from build123d import *

# Parameters (mm, degrees)
SKIZZE1_R                       = 6
AUFSATZ_LINEAR_AUSTRAGEN1_DEPTH = 5.5
SKIZZE2_R                       = 9
AUFSATZ_LINEAR_AUSTRAGEN2_DEPTH = 1
SKIZZE3_R                       = 2.5
SCHNITT_LINEAR_AUSTRAGEN1_DEPTH = 19.193405399
FASE1_SIZE                      = 0.2


with BuildPart() as part:
    # Skizze1 → Aufsatz-Linear austragen1 (new, symmetric)
    with BuildSketch(Plane.XY):
        Circle(SKIZZE1_R)
    extrude(amount=AUFSATZ_LINEAR_AUSTRAGEN1_DEPTH, both=True)

    # Skizze2 → Aufsatz-Linear austragen2 (add)
    with BuildSketch(Plane.XY.offset(5.5)):
        Circle(SKIZZE2_R)
    aufsatz_linear_austragen2 = extrude(amount=AUFSATZ_LINEAR_AUSTRAGEN2_DEPTH)

    # Spiegeln1: Aufsatz-Linear austragen2 across plane
    add(aufsatz_linear_austragen2.mirror(Plane.XY))

    # Skizze3 → Schnitt-Linear austragen1 (cut, through all)
    with BuildSketch(Plane(origin=(0, 0, -6.5), x_dir=(-1, 0, 0), z_dir=(0, 0, -1))):
        Circle(SKIZZE3_R)
    extrude(amount=-SCHNITT_LINEAR_AUSTRAGEN1_DEPTH, mode=Mode.SUBTRACT)

    # Fase1
    fase1_edges = [part.edges().sort_by_distance(p)[0] for p in [
        (-9, 0, -5.5),
        (2.5, 0, 6.5),
        (2.5, 0, -6.5),
        (-9, 0, 5.5),
        (-9, 0, 6.5),
        (-9, 0, -6.5),
    ]]
    chamfer(fase1_edges, length=FASE1_SIZE)


solid = part.part
The model under review builds one solid part; all positions refer to its coordinate system, in mm. A direction names the side the tool comes from. Round coordinates to 2 decimals unless told otherwise and drop trailing zeros. Order: outer loops, then holes, each group sorted by start corner. A loop starts at its lowest first (then second) coordinate and runs counter-clockwise, first axis right, second up. Notation, with made-up numbers: (-11.75, 5) -> (12.25, 5) arc R12 cw to (12.25, 11) -> close; hole circle Ø10 at (11.5, -11.75). An arc over 180 degrees is marked (long way). Write item = value, one per line. Start each with the question number.
Item 1: For faces 4 (the face through (-2.1, 2.1, 6.5)), 5 (the face through (2, -6, -5.5)), list the 3-axis set-ups (+Z, -Z, +X, -X, +Y, -Y) from which the entire face can be reached by the end or side of a thin tool; tool diameter is ignored.
Item 2: Consider section C-C on z = -4.5. Write out the cut boundary in (x, y).
Item 3: For line 1 along Z through (x, y) = (4.75, -4.75); line 2 along Y through (x, z) = (0, -2.75); line 3 along X through (y, z) = (0.75, 6), list the stretches that pass through material, from the lowest coordinate up.
Item 4: Consider section A-A on y = 0. Write out the cut boundary in (x, z), plus the area to 3 significant figures.
Item 5: Clearance check with flat-ended pins moving along their axes: pin 1 Ø1.5 at (x, z) = (-5.5, 1) entering from +Y; pin 2 Ø1.5 at (x, z) = (-1, -5) entering from -Y; pin 3 Ø1.5 at (y, z) = (-1.5, -5) entering from -X. State where each tip first meets the part, or that it passes through.
Item 6: Mouldability with a two-part tool opening along Y and no side actions: class faces 1 (the face through (0.54, -2.44, -0.09)), 2 (the face through (-6, 0, 0)), 3 (the face through (2, -6, 5.5)) as released by +Y, released by -Y, zero draft, split by the parting line, or undercut.
Conclusion:
q1.face_4 = +Z, +X, -X, +Y, -Y
q1.face_5 = none
q2.outline = circle Ø12 at (0, 0); hole circle Ø5 at (0, 0)
q3.line_1 = -6.5 to -5.5, 5.5 to 6.5
q3.line_2 = -6 to -2.5, 2.5 to 6
q3.line_3 = -8.97 to -2.38, 2.38 to 8.97
q4.outline = (-9, -6.3) -> (-8.8, -6.5) -> (-2.7, -6.5) -> (-2.5, -6.3) -> (-2.5, 6.3) -> (-2.7, 6.5) -> (-8.8, 6.5) -> (-9, 6.3) -> (-9, 5.7) -> (-8.8, 5.5) -> (-6, 5.5) -> (-6, -5.5) -> (-8.8, -5.5) -> (-9, -5.7) -> close; (2.5, -6.3) -> (2.7, -6.5) -> (8.8, -6.5) -> (9, -6.3) -> (9, -5.7) -> (8.8, -5.5) -> (6, -5.5) -> (6, 5.5) -> (8.8, 5.5) -> (9, 5.7) -> (9, 6.3) -> (8.8, 6.5) -> (2.7, 6.5) -> (2.5, 6.3) -> close
q4.area = 103 mm2
q5.pin_1 = 3.67
q5.pin_2 = -8.97
q5.pin_3 = -8.92
q6.face_1 = undercut
q6.face_2 = split by the parting line
q6.face_3 = zero draft
